```python
from build123d import *

# Parameters (mm, degrees)
SKETCH1_W           = 32
SKETCH1_H           = 32
BOSS_EXTRUDE1_DEPTH = 7


# Read off the part's stored shape, not the designer's step: AdvancedHole1
with BuildPart() as part:
    # Sketch1 → Boss-Extrude1 (new body)
    with BuildSketch(Plane(origin=(0, 0, 0), x_dir=(1, 0, 0), z_dir=(0, 1, 0))):
        Rectangle(SKETCH1_W, SKETCH1_H)
    extrude(amount=BOSS_EXTRUDE1_DEPTH)

    # AdvancedHole1 outline → AdvancedHole1 (revolve, cut)
    with BuildSketch(Plane(origin=(8, 0, 0), x_dir=(1, 0, 0), z_dir=(0, 0, 1))):
        Polygon((6.3, 4), (3.3, 4), (6.3, 7), (0, 7), (0, 0), (2.3, 0), align=None)
    revolve(axis=Axis((8, 0, 0), (0, 1, 0)), mode=Mode.SUBTRACT)

    # AdvancedHole1 2 outline → AdvancedHole1 2 (revolve, cut)
    with BuildSketch(Plane(origin=(-8, 0, 0), x_dir=(1, 0, 0), z_dir=(0, 0, 1))):
        Polygon((6.3, 4), (3.3, 4), (6.3, 7), (0, 7), (0, 0), (2.3, 0), align=None)
    revolve(axis=Axis((-8, 0, 0), (0, 1, 0)), mode=Mode.SUBTRACT)


solid = part.part
```
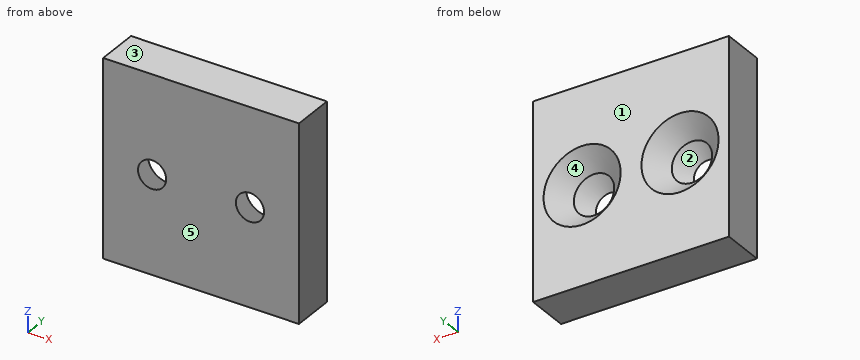
Part model, mm, in its own coordinate system. Face numbers are marked on the shaded views. A direction names the side the tool comes from. Give positions to 0.01 mm unless a question says otherwise; leave off trailing zeros. Loops run counter-clockwise (first coordinate to the right, second up) from the corner with the lowest first, then second, coordinate; pieces in that order, holes last. Notation, with made-up numbers: M 12,82.5 L 68,82.5 A30 cw 68,106.5 Z; hole C 22,48 d8. An arc over 180 degrees is marked long. Return JSON: item names as keys, results as strings.
1) Saw through at C-C, the plane y = 5. List the corners of the cut face in (x, z), then the cut area to 3 significant figures.
Calculated:
{"outline": "M -16,-16 L 16,-16 L 16,16 L -16,16 Z; hole C -8,0 d8.6; hole C 8,0 d8.6", "area": "908 mm2"}
2) Drill centre lines: line 1 (X direction, y = 2, z = -1.5); line 2 (Y direction, x = 4.5, z = -1); line 3 (Y direction, x = 8, z = 4.5). Where is each one in solid material? Low to high.
Calculated:
{"line 1": "x = -16 to -12.03, -3.97 to 3.97, 12.03 to 16", "line 2": "y = 0 to 1.34, 4 to 4.34", "line 3": "y = 0 to 2.2, 4 to 5.2"}
3) 3-axis set-ups, long thin cutter, end or side, ignore diameter. For the marked faces 1 and 2: which of +Z, -Z, +X, -X, +Y, -Y reach the whole face in a straight line?
Calculated:
{"face 1": "+Z, -Z, +X, -X, +Y", "face 2": "none"}
4) Pull direction Z, two halves, no side cores. Call the marked faces 3, 4 and 5: released by +Z, released by -Z, zero draft, split by the parting line, or undercut.
Calculated:
{"face 3": "released by +Z", "face 4": "undercut", "face 5": "zero draft"}
5) Saw through at A-A, the plane x = 8. List the corners of the cut face in (y, z), then the cut area to 3 significant figures.
Calculated:
{"outline": "M 0,-16 L 7,-16 L 7,-6.3 L 4,-3.3 L 4,-6.3 L 0,-2.3 Z; M 0,2.3 L 4,6.3 L 4,3.3 L 7,6.3 L 7,16 L 0,16 Z", "area": "161 mm2"}
6) Saw through at B-B, the plane z = 0. List the corners of the cut face in (x, y), then the cut area to 3 significant figures.
Calculated:
{"outline": "M -16,0 L -10.3,0 L -14.3,4 L -11.3,4 L -14.3,7 L -16,7 Z; M -5.7,0 L 5.7,0 L 1.7,4 L 4.7,4 L 1.7,7 L -1.7,7 L -4.7,4 L -1.7,4 Z; M 10.3,0 L 16,0 L 16,7 L 14.3,7 L 11.3,4 L 14.3,4 Z", "area": "97.6 mm2"}
7) Flat gauge pin, fed straight in: pin 1 Ø4 at (x, z) = (5.5, 2.5) entering from -Y. Where does the tip first touch, or does it go through?
Calculated:
{"pin 1": "stops at y = 0"}
8) Saw through at D-D, the plane y = 2.5. List the corners of the cut face in (x, z), then the cut area to 3 significant figures.
Calculated:
{"outline": "M -16,-16 L 16,-16 L 16,16 L -16,16 Z; hole C -8,0 d9.6; hole C 8,0 d9.6", "area": "879 mm2"}
